from build123d import *

# Parameters (mm, degrees)
BOSS_EXTRUDE2_DEPTH = 10


with BuildPart() as part:
    # Sketch1 → Boss-Extrude2 (new body)
    with BuildSketch(Plane(origin=(0, 0, 0), x_dir=(0, 1, 0), z_dir=(0, 0, 1))):
        with BuildLine():
            Line((21.3, 83), (21.3, 92.9))
            ThreePointArc((21.3, 92.9), (21.270710678, 92.970710678), (21.2, 93))
            Line((21.2, 93), (2.8, 93))
            ThreePointArc((2.8, 93), (2.729289322, 92.970710678), (2.7, 92.9))
            Line((2.7, 92.9), (2.7, 83))
            ThreePointArc((2.7, 83), (3.234857225, 80.75), (4.725, 78.981371503))
            ThreePointArc((4.725, 78.981371503), (6.215142775, 77.212743005), (6.75, 74.962743005))
            Line((6.75, 74.962743005), (6.75, 68.356371503))
            ThreePointArc((6.75, 68.356371503), (5.871320344, 66.235051159), (3.75, 65.356371503))
            Line((3.75, 65.356371503), (-2.25, 65.356371503))
            ThreePointArc((-2.25, 65.356371503), (-4.371320344, 64.477691846), (-5.25, 62.356371503))
            Line((-5.25, 62.356371503), (-5.25, 45.25))
            ThreePointArc((-5.25, 45.25), (-5.909009742, 43.659009742), (-7.5, 43))
            ThreePointArc((-7.5, 43), (-8.914213562, 42.414213562), (-9.5, 41))
            Line((-9.5, 41), (-9.5, 2))
            ThreePointArc((-9.5, 2), (-8.914213562, 0.585786438), (-7.5, 0))
            Line((-7.5, 0), (7.5, 0))
            ThreePointArc((7.5, 0), (8.914213562, 0.585786438), (9.5, 2))
            Line((9.5, 2), (9.5, 41))
            ThreePointArc((9.5, 41), (8.914213562, 42.414213562), (7.5, 43))
            ThreePointArc((7.5, 43), (5.909009742, 43.659009742), (5.25, 45.25))
            Line((5.25, 45.25), (5.25, 51.856371503))
            ThreePointArc((5.25, 51.856371503), (6.128679656, 53.977691846), (8.25, 54.856371503))
            Line((8.25, 54.856371503), (14.25, 54.856371503))
            ThreePointArc((14.25, 54.856371503), (16.371320344, 55.735051159), (17.25, 57.856371503))
            Line((17.25, 57.856371503), (17.25, 74.962743005))
            ThreePointArc((17.25, 74.962743005), (17.784857225, 77.212743005), (19.275, 78.981371503))
            ThreePointArc((19.275, 78.981371503), (20.765142775, 80.75), (21.3, 83))
        make_face()
    extrude(amount=BOSS_EXTRUDE2_DEPTH)


solid = part.part
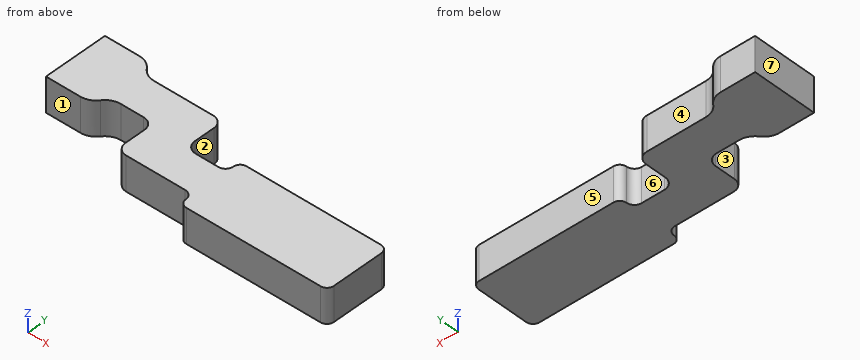
For this review, take the finished solid that the model builds, in its own axes (mm). Face numbers are marked on the shaded views. A direction names the side the tool comes from. Coordinates: 2 decimals unless noted, no trailing zeros. Order: outer loops, then holes, each group sorted by start corner. A loop starts at its lowest first (then second) coordinate and runs counter-clockwise, first axis right, second up. Notation, with made-up numbers: (84, 2.25) - (99, 2.25) arc R10 cw to (99, 18.25) - close; hole circle Ø10 at (83.5, 32). An arc over 180 degrees is marked (long way). Use one line per item in the form item = value.
Q1. For P1, Ø6, axis at x = -42.5, z = 5, coming from the +Y side; P2, Ø2, axis at x = -73, z = 7.5, coming from the -Y side; P3, Ø4, axis at y = 5.5, z = 1.5, coming from the +X side; P4, Ø5, axis at x = -88, z = 5, coming from the -Y side, all flat-tipped, find the tip position at first contact; note any pin that passes through.
Checked values:
P1 = 9.5
P2 = 6.75
P3 = 0
P4 = 2.7
Q2. For probe 1 along Y at (x, z) = (-85.5, 4.75); probe 2 along Y at (x, z) = (-25, 4); probe 3 along X at (y, z) = (10, 4), list the stretches that pass through material, from the lowest coordinate up. Write a range as from..to.
Checked values:
probe_1 = 2.7..21.3
probe_2 = -9.5..9.5
probe_3 = -93..-54.86
Q3. Consider section A-A (z = 1.75). Give the boundary of the cut face in (x, y) (3 decimals).
Checked values:
outline = (-93, 2.8) arc R0.1 ccw to (-92.9, 2.7) - (-83, 2.7) arc R5 ccw to (-78.981, 4.725) arc R5 cw to (-74.963, 6.75) - (-68.356, 6.75) arc R3 cw to (-65.356, 3.75) - (-65.356, -2.25) arc R3 ccw to (-62.356, -5.25) - (-45.25, -5.25) arc R2.25 cw to (-43, -7.5) arc R2 ccw to (-41, -9.5) - (-2, -9.5) arc R2 ccw to (0, -7.5) - (0, 7.5) arc R2 ccw to (-2, 9.5) - (-41, 9.5) arc R2 ccw to (-43, 7.5) arc R2.25 cw to (-45.25, 5.25) - (-51.856, 5.25) arc R3 cw to (-54.856, 8.25) - (-54.856, 14.25) arc R3 ccw to (-57.856, 17.25) - (-74.963, 17.25) arc R5 cw to (-78.981, 19.275) arc R5 ccw to (-83, 21.3) - (-92.9, 21.3) arc R0.1 ccw to (-93, 21.2) - close
Q4. Draft analysis for pull direction X (two halves, no side actions). For the marked faces 5, 6 and 7, state which applies: +X half, -X half, draft (parallel to the pull), parting line (faces both ways), or undercut.
Checked values:
face_5 = draft
face_6 = undercut
face_7 = -X half
Q5. Consider section C-C (y = 1.5). Give the boundary of the cut face in (x, z).
Checked values:
outline = (-65.36, 0) - (0, 0) - (0, 10) - (-65.36, 10) - close
Q6. For the marked faces 1, 2, 3 and 4, list the 3-axis set-ups (+Z, -Z, +X, -X, +Y, -Y) from which the entire face can be reached by the end or side of a thin tool; tool diameter is ignored.
Checked values:
face_1 = +Z, -Z, -X, -Y
face_2 = +Z, -Z, +Y
face_3 = +Z, -Z, -Y
face_4 = +Z, -Z, +X, +Y
Q7. Consider section B-B (x = -31). Give the boundary of the cut face in (y, z), then the cut area to 3 significant figures.
Checked values:
outline = (-9.5, 0) - (9.5, 0) - (9.5, 10) - (-9.5, 10) - close
area = 190 mm2
